Answer from the drawing. Dimensions are ordinates in mm from the lowest x, y and z of the part. A direction names the side the tool comes from. Round coordinates to 2 decimals unless told otherwise and drop trailing zeros. Loops run counter-clockwise (first coordinate to the right, second up) from the corner with the lowest first, then second, coordinate; pieces in that order, holes last. Notation, with made-up numbers: M 68.25,-29 L 111.25,-29 A21 cw 111.25,9 Z; hole C 6,-9.75 d6. An arc over 180 degrees is marked long. Answer as a JSON object with one key per item and string values.
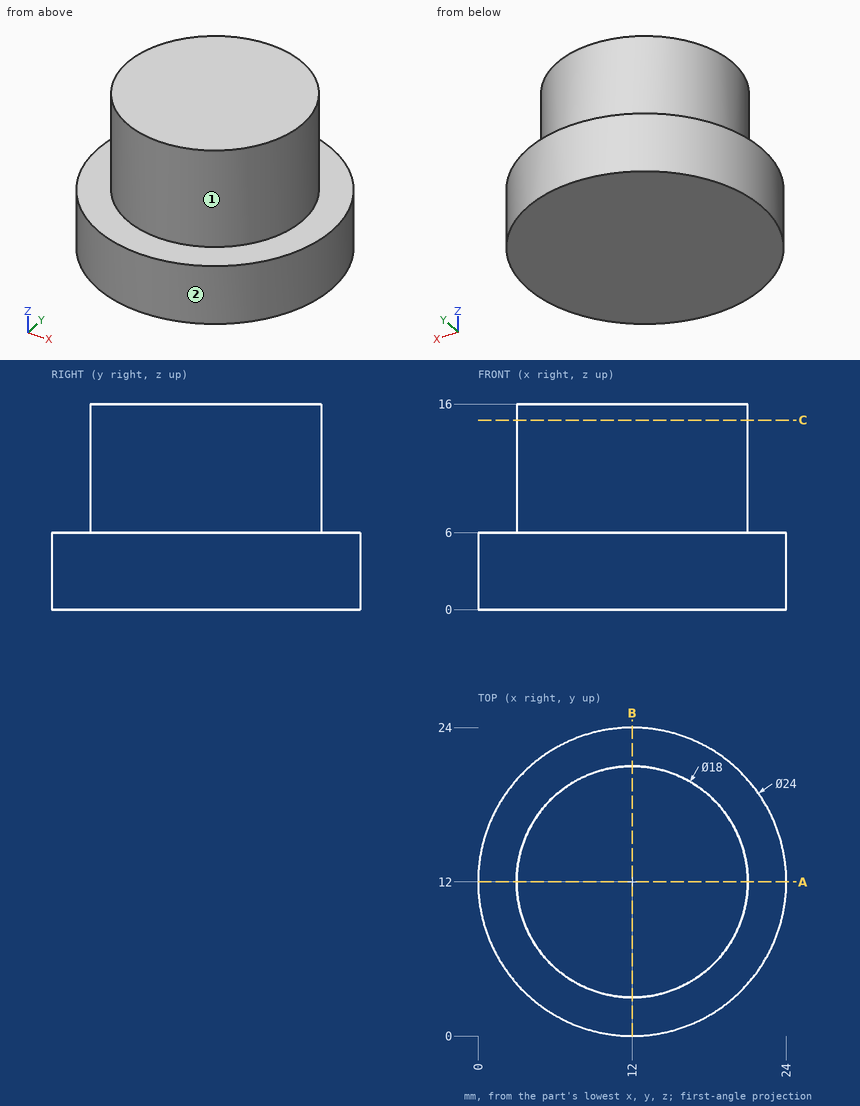
Item 1: Straight lines are drawn through the part: line 1 (X direction, y = 12.25, z = 13.5); line 2 (Z direction, x = 2.5, y = 8.75); line 3 (X direction, y = 9, z = 13.25). For each, find the intervals that lie inside material, in ascending order.
Values follow:
{"line 1": "3 to 21", "line 2": "0 to 6", "line 3": "3.51 to 20.49"}
Item 2: Flat-ended cylindrical pins translate along their axes: P1, Ø8, axis at y = 17.5, z = 14.5, coming from the +X side; P2, Ø2, axis at y = 8, z = 6.5, coming from the -X side; P3, Ø1, axis at y = 12, z = 8.5, coming from the +X side. Find the tip coordinate at first contact, or state that the pin passes through.
Values follow:
{"P1": "x = 20.87", "P2": "x = 0.42", "P3": "x = 21"}
Item 3: The part is cut by section C-C (z = 14.75). Give the vertices of the cut face in (x, y), then the cut area to 3 significant figures.
Values follow:
{"outline": "C 12,12 d18", "area": "254 mm^2"}
Item 4: The part is cut by section A-A (y = 12). Give the vertices of the cut face in (x, z).
Values follow:
{"outline": "M 0,0 L 24,0 L 24,6 L 21,6 L 21,16 L 3,16 L 3,6 L 0,6 Z"}
Item 5: Which of the six approach directions +Z, -Z, +X, -X, +Y, -Y give full straight-line access (tool end or side, diameter ignored) to the marked faces 1 and 2?
Values follow:
{"face 1": "+Z", "face 2": "+Z, -Z"}
